Design review of the part shown in the three views and the two pictorial views. Dimensions are in mm from the part's minimum x, y and z. A direction names the side the tool comes from. Give positions to 0.01 mm unless a question says otherwise; leave off trailing zeros. Order: outer loops, then holes, each group sorted by start corner. A loop starts at its lowest first (then second) coordinate and runs counter-clockwise, first axis right, second up. Notation, with made-up numbers: M 30.5,9.25 L 46.5,9.25 A23 cw 46.5,17.25 Z; hole C 30,-32.75 d3. An arc over 180 degrees is marked long. Answer as a JSON object with one key per item and string values.
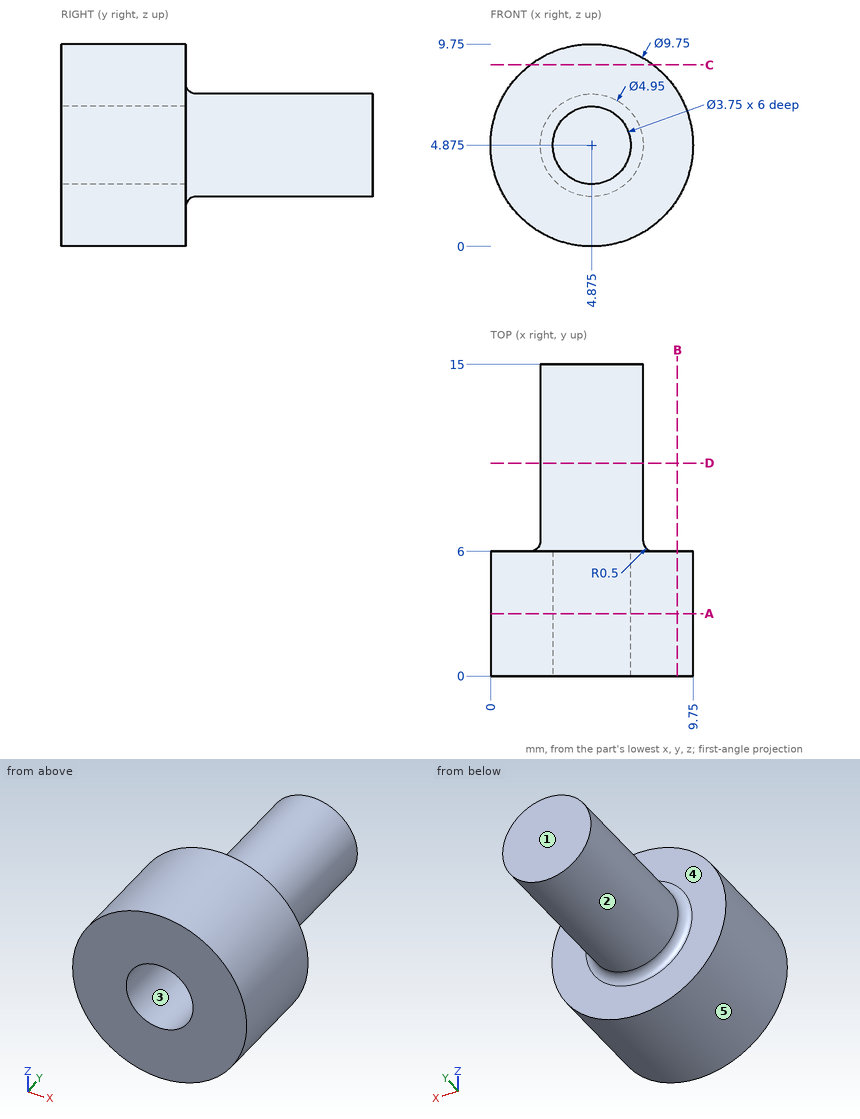
(1) To check wall thickness, follow L1, parallel to Y at x = 9, z = 4.5; L2, parallel to X at y = 4.25, z = 4.25; L3, parallel to X at y = 7.75, z = 5. State the ranges of each line that lie inside material, in increasing order. Write a range as from..to.
Checked values:
{"L1": "y = 0..6", "L2": "x = 0.04..3.11, 6.64..9.71", "L3": "x = 2.4..7.35"}
(2) Draft analysis for pull direction X (two halves, no side actions). For the marked faces 1, 2 and 3, state which applies: +X half, -X half, draft (parallel to the pull), parting line (faces both ways), or undercut.
Checked values:
{"face 1": "draft", "face 2": "parting line", "face 3": "undercut"}
(3) We need section C-C (z = 8.75). Write out the cut boundary in (x, y).
Checked values:
{"outline": "M 1.92,0 L 7.83,0 L 7.83,6 L 1.92,6 Z"}
(4) We need section D-D (y = 10.25). Write out the cut boundary in (x, z) (3 decimals), plus the area to 3 significant figures.
Checked values:
{"outline": "C 4.875,4.875 d4.95", "area": "19.2 mm^2"}
(5) We need section A-A (y = 3). Write out the cut boundary in (x, z) (3 decimals), plus the area to 3 significant figures.
Checked values:
{"outline": "C 4.875,4.875 d9.75; hole C 4.875,4.875 d3.75", "area": "63.6 mm^2"}
(6) Insertion check: pin 1 (1.9 mm diameter, centred on x = 5, z = 4.5, fed in from -Y); pin 2 (2 mm diameter, centred on y = 11, z = 7.5, fed in from +X); pin 3 (3 mm diameter, centred on y = 6, z = 7, fed in from +X). Each pin has a flat end and moves straight along its axis. Give the tip position at first contact, or say it passes through.
Checked values:
{"pin 1": "stops at y = 6", "pin 2": "stops at x = 6.74", "pin 3": "stops at x = 9.71"}
(7) We need section B-B (x = 9). Write out the cut boundary in (y, z).
Checked values:
{"outline": "M 0,2.28 L 6,2.28 L 6,7.47 L 0,7.47 Z"}
(8) Tool access review of the marked faces 4 and 5: name each direction out of +Z, -Z, +X, -X, +Y, -Y from which nothing blocks a thin tool from reaching the whole face with its end or side.
Checked values:
{"face 4": "+Y", "face 5": "+Y, -Y"}
